```python
from build123d import *

# Parameters (mm, degrees)
REVOLVE2_ANGLE     = 270
CUT_EXTRUDE1_REACH = 141
CUT_EXTRUDE2_REACH = 122
SKETCH3_R          = 3.75
CUT_EXTRUDE3_DEPTH = 41
CUT_EXTRUDE4_DEPTH = 10
FILLET1_R          = 1


with BuildPart() as part:
    # Sketch1 → Revolve2 (revolve)
    with BuildSketch(Plane(origin=(0, 0, 0), x_dir=(1, 0, 0), z_dir=(0, 1, 0))):
        with BuildLine():
            Line((0, 0), (0, 25))
            Line((0, 25), (17, 25))
            ThreePointArc((17, 25), (18.414213562, 25.585786438), (19, 27))
            Line((19, 27), (19, 40))
            Line((19, 40), (47.5, 40))
            Line((47.5, 40), (50, 37.5))
            Line((50, 37.5), (89, 37.5))
            Line((89, 37.5), (91.5, 40))
            Line((91.5, 40), (120, 40))
            Line((120, 40), (120, 27))
            ThreePointArc((120, 27), (120.585786438, 25.585786438), (122, 25))
            Line((122, 25), (139, 25))
            Line((139, 25), (139, 0))
            Line((139, 0), (0, 0))
        make_face()
    revolve(axis=Axis((139, 0, 0), (-1, 0, 0)), revolution_arc=REVOLVE2_ANGLE)

    # Sketch2 → Cut-Extrude1 (cut, up to next)
    with BuildSketch(Plane(origin=(139, 0, 0), x_dir=(0, 0, -1), z_dir=(1, 0, 0)), mode=Mode.PRIVATE) as cut_extrude1_sk1:
        with BuildLine():
            Line((-12, 4), (0, 4))
            Line((0, 4), (0, 10))
            Line((0, 10), (-12, 10))
            ThreePointArc((-12, 10), (-15, 7), (-12, 4))
        make_face()
    cut_extrude1_tool1 = extrude(cut_extrude1_sk1.sketch, amount=-CUT_EXTRUDE1_REACH, mode=Mode.PRIVATE) & part.part
    add(cut_extrude1_tool1.solids().sort_by_distance((139, 7, 7.193712))[0], mode=Mode.SUBTRACT)

    # Sketch3 → Cut-Extrude2 (cut, up to next)
    with BuildSketch(Plane(origin=(120, 0, 0), x_dir=(0, 0, -1), z_dir=(1, 0, 0)), mode=Mode.PRIVATE) as cut_extrude2_sk1:
        with Locations((-8.783194418, 30.77101714)):
            Circle(SKETCH3_R)
    cut_extrude2_tool1 = extrude(cut_extrude2_sk1.sketch, amount=-CUT_EXTRUDE2_REACH, mode=Mode.PRIVATE) & part.part
    add(cut_extrude2_tool1.solids().sort_by_distance((120, 30.771017, 8.783194))[0], mode=Mode.SUBTRACT)
    # Sketch3 → Cut-Extrude2 (cut, up to next)
    with BuildSketch(Plane(origin=(120, 0, 0), x_dir=(0, 0, -1), z_dir=(1, 0, 0)), mode=Mode.PRIVATE) as cut_extrude2_sk2:
        with Locations((31.040079752, -7.779039077)):
            Circle(SKETCH3_R)
    cut_extrude2_tool2 = extrude(cut_extrude2_sk2.sketch, amount=-CUT_EXTRUDE2_REACH, mode=Mode.PRIVATE) & part.part
    add(cut_extrude2_tool2.solids().sort_by_distance((120, -7.779039, -31.04008))[0], mode=Mode.SUBTRACT)
    # Sketch3 → Cut-Extrude2 (cut, up to next)
    with BuildSketch(Plane(origin=(120, 0, 0), x_dir=(0, 0, -1), z_dir=(1, 0, 0)), mode=Mode.PRIVATE) as cut_extrude2_sk3:
        with Locations((18.777810674, -25.911268327)):
            Circle(SKETCH3_R)
    cut_extrude2_tool3 = extrude(cut_extrude2_sk3.sketch, amount=-CUT_EXTRUDE2_REACH, mode=Mode.PRIVATE) & part.part
    add(cut_extrude2_tool3.solids().sort_by_distance((120, -25.911268, -18.777811))[0], mode=Mode.SUBTRACT)
    # Sketch3 → Cut-Extrude2 (cut, up to next)
    with BuildSketch(Plane(origin=(120, 0, 0), x_dir=(0, 0, -1), z_dir=(1, 0, 0)), mode=Mode.PRIVATE) as cut_extrude2_sk4:
        with Locations((-2.270804711, -31.919327154)):
            Circle(SKETCH3_R)
    cut_extrude2_tool4 = extrude(cut_extrude2_sk4.sketch, amount=-CUT_EXTRUDE2_REACH, mode=Mode.PRIVATE) & part.part
    add(cut_extrude2_tool4.solids().sort_by_distance((120, -31.919327, 2.270805))[0], mode=Mode.SUBTRACT)
    # Sketch3 → Cut-Extrude2 (cut, up to next)
    with BuildSketch(Plane(origin=(120, 0, 0), x_dir=(0, 0, -1), z_dir=(1, 0, 0)), mode=Mode.PRIVATE) as cut_extrude2_sk5:
        with Locations((-22.256885334, -22.991978062)):
            Circle(SKETCH3_R)
    cut_extrude2_tool5 = extrude(cut_extrude2_sk5.sketch, amount=-CUT_EXTRUDE2_REACH, mode=Mode.PRIVATE) & part.part
    add(cut_extrude2_tool5.solids().sort_by_distance((120, -22.991978, 22.256885))[0], mode=Mode.SUBTRACT)
    # Sketch3 → Cut-Extrude2 (cut, up to next)
    with BuildSketch(Plane(origin=(120, 0, 0), x_dir=(0, 0, -1), z_dir=(1, 0, 0)), mode=Mode.PRIVATE) as cut_extrude2_sk6:
        with Locations((-31.828721952, -3.306426908)):
            Circle(SKETCH3_R)
    cut_extrude2_tool6 = extrude(cut_extrude2_sk6.sketch, amount=-CUT_EXTRUDE2_REACH, mode=Mode.PRIVATE) & part.part
    add(cut_extrude2_tool6.solids().sort_by_distance((120, -3.306427, 31.828722))[0], mode=Mode.SUBTRACT)
    # Sketch3 → Cut-Extrude2 (cut, up to next)
    with BuildSketch(Plane(origin=(120, 0, 0), x_dir=(0, 0, -1), z_dir=(1, 0, 0)), mode=Mode.PRIVATE) as cut_extrude2_sk7:
        with Locations((-26.507545832, 17.926238144)):
            Circle(SKETCH3_R)
    cut_extrude2_tool7 = extrude(cut_extrude2_sk7.sketch, amount=-CUT_EXTRUDE2_REACH, mode=Mode.PRIVATE) & part.part
    add(cut_extrude2_tool7.solids().sort_by_distance((120, 17.926238, 26.507546))[0], mode=Mode.SUBTRACT)

    # Sketch4 → Cut-Extrude3 (cut, through all)
    with BuildSketch(Plane(origin=(0, 0, 0), x_dir=(1, 0, 0), z_dir=(0, 1, 0))):
        with BuildLine():
            Line((0, 40), (0, 10))
            ThreePointArc((0, 10), (2.614672282, 10.114159057), (5.20944533, 10.45576741))
            Line((5.20944533, 10.45576741), (6.077686218, 5.531728645))
            ThreePointArc((6.077686218, 5.531728645), (23.263426891, 13.850182233), (33.526230894, 29.950530259))
            Line((33.526230894, 29.950530259), (28.938382586, 32.089879059))
            ThreePointArc((28.938382586, 32.089879059), (29.733411153, 36.00947858), (30, 40))
            Line((30, 40), (0, 40))
        make_face()
    extrude(amount=-CUT_EXTRUDE3_DEPTH, mode=Mode.SUBTRACT)

    # Sketch5 → Cut-Extrude4 (cut)
    with BuildSketch(Plane(origin=(139, 0, 0), x_dir=(0, 0, -1), z_dir=(1, 0, 0))):
        with BuildLine():
            Line((-4, 0), (-12, 0))
            Line((-12, 0), (-21, 0))
            ThreePointArc((-21, 0), (-2.009217424, -20.903661051), (20.615528128, -4))
            Line((20.615528128, -4), (0, -4))
            Line((0, -4), (-4, -4))
            Line((-4, -4), (-4, 0))
        make_face()
    extrude(amount=-CUT_EXTRUDE4_DEPTH, mode=Mode.SUBTRACT)

    # Fillet1
    fillet1_edges = [part.edges().sort_by_distance(p)[0] for p in [
        (129, 0, 12.5),
        (129, -4, -8.307764064),
        (129, -20.903661051, 2.009217424),
        (129, -2, 4),
    ]]
    fillet(fillet1_edges, radius=FILLET1_R)


solid = part.part
```
Here's how the part is built. I have some questions about the finished solid (model axes, mm). A direction names the side the tool comes from. Give positions to 0.01 mm unless a question says otherwise; leave off trailing zeros. Order: outer loops, then holes, each group sorted by start corner. A loop starts at its lowest first (then second) coordinate and runs counter-clockwise, first axis right, second up. Notation, with made-up numbers: (62, -32) -> (96, -32) arc R26 cw to (96, -7) -> close; hole circle Ø3 at (42, 83). An arc over 180 degrees is marked (long way). Use CSV: the item, a comma, the result in double quotes. Start each with the question number.
Item 1: If I drill on probe 1 along Y at (x, z) = (55.5, 10.5); probe 2 along Z at (x, y) = (114, 18); probe 3 along X at (y, z) = (20.5, 21), over which ranges is the centre line in solid material (lowest first)? Write a range as [from, to].
Item 2: On a 3-axis mill with a long thin cutter (end or side, diameter ignored), from which of +Z, -Z, +X, -X, +Y, -Y can I reach the whole of each face in a straight line? I mean faces 1 (the flat face through (70, 10, 6)), 2 (the flat face through (86, 0, -16)), 3 (the flat face through (135, -4, -8)), 4 (the conical face through (49.879, -27.465, 25.711)), 5 (the cylindrical face through (23.06, -14.73, -13.67)). Say none if no direction works.
Item 3: Suppose I cut it at D-D (x = 65). List the corners of the cut face in (y, z) for me, and give its area (3 significant figures).
Item 4: Suppose I cut it at B-B (x = 27.5). List the corners of the cut face in (y, z) for me.
Item 5: Suppose I cut it at A-A (x = 101). List the corners of the cut face in (y, z) for me.
Item 6: I'm going to push flat-ended pins straight in: P1, Ø10, axis at y = -3.31, z = 31.83, coming from the -X side; P2, Ø12, axis at x = 51.5, z = 21, coming from the -Y side; P3, Ø12, axis at x = 80.5, z = -14.5, coming from the +Y side. Where does each tip first touch, or does it pass through?
Item 7: Suppose I cut it at C-C (x = 13). List the corners of the cut face in (y, z) for me.
Item 8: Thinking about a two-plate mould opening in Y: for faces 6 (the flat face through (5.637, -12.019, -8.028)), 7 (the cylindrical face through (70.21, 14.6, 24.78)), 8 (the cylindrical face through (130.619, -18.251, 17.085)), which applies, pulls with the +Y half, pulls with the -Y half, needs draft (parallel to the pull), parting line crosses it, or undercut?
Answer block:
1,probe 1,"y = [-36, 4], [10, 27.44], [34.1, 36]"
1,probe 2,"z = [0, 22.76], [30.26, 35.72]"
1,probe 3,"x = [19, 120]"
2,face 1,"-Z, +X, -X"
2,face 2,"-Z, +X, -X, +Y"
2,face 3,"+X"
2,face 4,"none"
2,face 5,"+Y, -Y"
3,outline,"(0, -37.5) -> (0, 0) -> (4, 0) -> (4, 12) arc R3 cw to (10, 12) -> (10, 0) -> (37.5, 0) arc R37.5 ccw (long way) to start; hole circle Ø7.5 at (-31.92, 2.27); hole circle Ø7.5 at (-25.91, -18.78); hole circle Ø7.5 at (-22.99, 22.26); hole circle Ø7.5 at (-7.78, -31.04); hole circle Ø7.5 at (-3.31, 31.83); hole circle Ø7.5 at (17.93, 26.51); hole circle Ø7.5 at (30.77, 8.78)"
3,area,"2,920 mm^2"
4,outline,"(-35.54, -18.35) -> (-29.64, -18.35) arc R3.75 cw to (-22.19, -18.35) -> (0, -18.35) -> (0, 0) -> (4, 0) -> (4, 12) arc R3 cw to (10, 12) -> (10, 0) -> (40, 0) arc R40 ccw (long way) to start; hole circle Ø7.5 at (-31.92, 2.27); hole circle Ø7.5 at (-22.99, 22.26); hole circle Ø7.5 at (-3.31, 31.83); hole circle Ø7.5 at (17.93, 26.51); hole circle Ø7.5 at (30.77, 8.78)"
5,outline,"(0, -40) -> (0, 0) -> (4, 0) -> (4, 12) arc R3 cw to (10, 12) -> (10, 0) -> (40, 0) arc R40 ccw (long way) to start; hole circle Ø7.5 at (-31.92, 2.27); hole circle Ø7.5 at (-25.91, -18.78); hole circle Ø7.5 at (-22.99, 22.26); hole circle Ø7.5 at (-7.78, -31.04); hole circle Ø7.5 at (-3.31, 31.83); hole circle Ø7.5 at (17.93, 26.51); hole circle Ø7.5 at (30.77, 8.78)"
6,P1,"stops at x = 19"
6,P2,"stops at y = -36.43"
6,P3,"stops at y = 0"
7,outline,"(-23.85, -7.5) -> (0, -7.5) -> (0, 0) -> (4, 0) -> (4, 12) arc R3 cw to (10, 12) -> (10, 0) -> (25, 0) arc R25 ccw (long way) to start"
8,face 6,"needs draft"
8,face 7,"undercut"
8,face 8,"parting line crosses it"
